Could you check a few things on this drawing? It's one solid part, dimensions in mm from its lowest x, y, z. Round coordinates to 2 decimals unless told otherwise and drop trailing zeros. Loops run counter-clockwise (first coordinate to the right, second up) from the corner with the lowest first, then second, coordinate; pieces in that order, holes last. Notation, with made-up numbers: (-40, 82.25) -> (-29, 82.25) arc R24 ccw to (-29, 118.25) -> close; hole circle Ø1 at (17.5, -7.5). An arc over 180 degrees is marked (long way). Write each question's results on one line, items separated by ' | '.
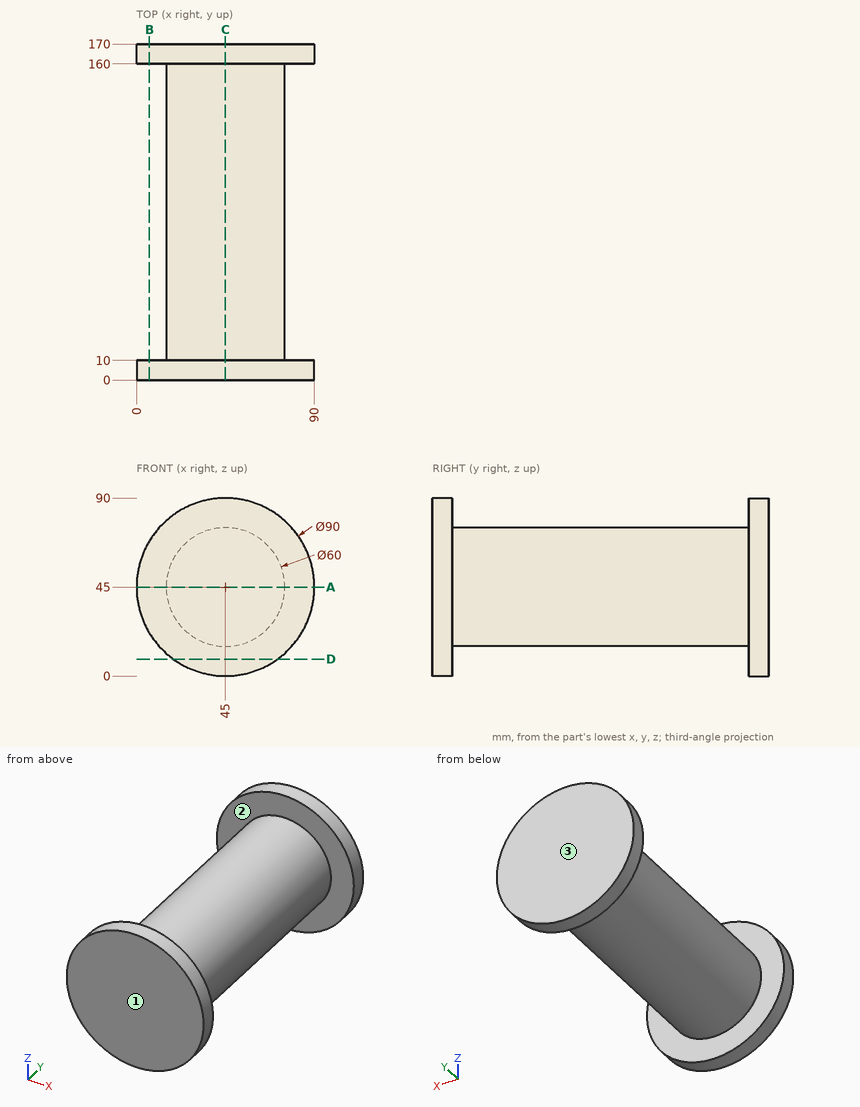
1) I'm going to push flat-ended pins straight in: pin 1 (5 mm diameter, centred on y = 65, z = 43.5, fed in from +X); pin 2 (1 mm diameter, centred on y = 61, z = 68.5, fed in from -X); pin 3 (2 mm diameter, centred on x = 18, z = 78.5, fed in from -Y); pin 4 (8 mm diameter, centred on x = 80, y = 40.5, fed in from -Z). Where does each tip first touch, or does it pass through?
Model answer:
pin 1: stops at x = 75 | pin 2: stops at x = 25.74 | pin 3: stops at y = 0 | pin 4: passes through
2) I need wall thicknesses on line 1 (Y direction, x = 8, z = 41); line 2 (X direction, y = 149, z = 44); line 3 (X direction, y = 66, z = 49). Which ranges of each line are inside material? Lowest first, please.
Model answer:
line 1: y = 0 to 10, 160 to 170 | line 2: x = 15.02 to 74.98 | line 3: x = 15.27 to 74.73
3) I want a section at B-B, the plane x = 6.5. Write out the boundary of the cut face in (y, z), plus the area to 3 significant figures.
Model answer:
outline: (0, 21.7) -> (10, 21.7) -> (10, 68.3) -> (0, 68.3) -> close; (160, 21.7) -> (170, 21.7) -> (170, 68.3) -> (160, 68.3) -> close | area: 932 mm2
4) I want a section at D-D, the plane z = 8.5. Write out the boundary of the cut face in (x, y), plus the area to 3 significant figures.
Model answer:
outline: (18.68, 0) -> (71.32, 0) -> (71.32, 10) -> (18.68, 10) -> close; (18.68, 160) -> (71.32, 160) -> (71.32, 170) -> (18.68, 170) -> close | area: 1,050 mm2
5) If we mould it in two halves opening along Y, with no side actions, what happens to the marked faces 1, 2 and 3? For each: released by +Y, released by -Y, zero draft, split by the parting line, or undercut.
Model answer:
face 1: released by -Y | face 2: undercut | face 3: released by +Y
6) I want a section at A-A, the plane z = 45. Write out the boundary of the cut face in (x, y), plus the area to 3 significant figures.
Model answer:
outline: (0, 0) -> (90, 0) -> (90, 10) -> (75, 10) -> (75, 160) -> (90, 160) -> (90, 170) -> (0, 170) -> (0, 160) -> (15, 160) -> (15, 10) -> (0, 10) -> close | area: 10,800 mm2
7) I want a section at C-C, the plane x = 45. Write out the boundary of the cut face in (y, z), plus the area to 3 significant figures.
Model answer:
outline: (0, 0) -> (10, 0) -> (10, 15) -> (160, 15) -> (160, 0) -> (170, 0) -> (170, 90) -> (160, 90) -> (160, 75) -> (10, 75) -> (10, 90) -> (0, 90) -> close | area: 10,800 mm2
